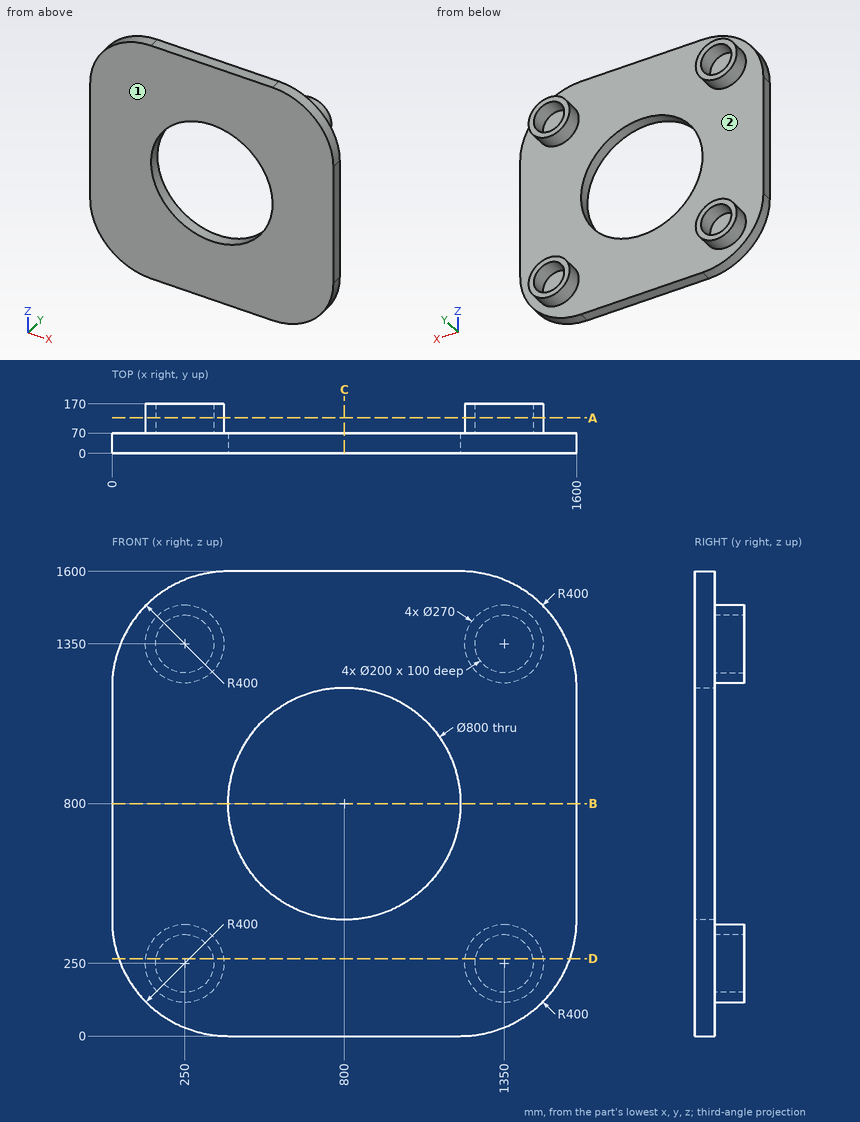
Geometry: see drawing. Coordinates: mm, zero at the bounding-box minimum. Coordinates: 2 decimals unless noted, no trailing zeros. Loops run counter-clockwise (first coordinate to the right, second up) from the corner with the lowest first, then second, coordinate; pieces in that order, holes last. Notation, with made-up numbers: (6, 87) -> (26, 87) arc R18 cw to (26, 118) -> close; hole circle Ø3 at (69, 64.5). An arc over 180 degrees is marked (long way). Use a Markdown table: item, result.
1) Cut plane C-C (x = 800). Return the cut outline in (y, z).
Results found:
| item | result |
|---|---|
| outline | (0, 0) -> (70, 0) -> (70, 400) -> (0, 400) -> close; (0, 1200) -> (70, 1200) -> (70, 1600) -> (0, 1600) -> close |
2) Cut plane D-D (z = 266.5). Return the cut outline in (x, y), then the cut area to 3 significant figures.
Results found:
| item | result |
|---|---|
| outline | (22.94, 0) -> (1577.06, 0) -> (1577.06, 70) -> (1483.99, 70) -> (1483.99, 170) -> (1448.63, 170) -> (1448.63, 70) -> (1251.37, 70) -> (1251.37, 170) -> (1216.01, 170) -> (1216.01, 70) -> (383.99, 70) -> (383.99, 170) -> (348.63, 170) -> (348.63, 70) -> (151.37, 70) -> (151.37, 170) -> (116.01, 170) -> (116.01, 70) -> (22.94, 70) -> close |
| area | 123,000 mm2 |
3) Cut plane A-A (y = 122). Return the cut outline in (x, z).
Results found:
| item | result |
|---|---|
| outline | circle Ø270 at (250, 250); circle Ø270 at (250, 1350); circle Ø270 at (1350, 250); circle Ø270 at (1350, 1350); hole circle Ø200 at (250, 250); hole circle Ø200 at (250, 1350); hole circle Ø200 at (1350, 250); hole circle Ø200 at (1350, 1350) |
4) Cut plane B-B (z = 800). Return the cut outline in (x, y), then the cut area to 3 significant figures.
Results found:
| item | result |
|---|---|
| outline | (0, 0) -> (400, 0) -> (400, 70) -> (0, 70) -> close; (1200, 0) -> (1600, 0) -> (1600, 70) -> (1200, 70) -> close |
| area | 56,000 mm2 |
5) Pull-direction query (X, two-part tool) for the marked faces 1 and 2; classes: released by +X, released by -X, zero draft, split by the parting line, or undercut.
Results found:
| item | result |
|---|---|
| face 1 | zero draft |
| face 2 | undercut |
6) Contact query for flat-ended pins moving along their axis: pin 1 (1 mm diameter, centred on y = 93, z = 1242, fed in from -X); pin 2 (10 mm diameter, centred on y = 107.5, z = 1313, fed in from -X); pin 3 (12 mm diameter, centred on x = 1222.5, y = 117.5, fed in from -Z). Output: stop coordinate, or through.
Results found:
| item | result |
|---|---|
| pin 1 | stops at x = 168.34 |
| pin 2 | stops at x = 118.85 |
| pin 3 | stops at z = 191.15 |
7) Material intervals for line 1 along X through (y, z) = (128, 1350); line 2 along Z through (x, y) = (1375, 74) (3 decimals); line 3 along X through (y, z) = (98, 268), sorted ascending. Write a range as from..to.
Results found:
| item | result |
|---|---|
| line 1 | x = 115..150, 350..385, 1215..1250, 1450..1485 |
| line 2 | z = 117.335..153.175, 346.825..382.665, 1217.335..1253.175, 1446.825..1482.665 |
| line 3 | x = 116.21..151.63, 348.37..383.79, 1216.21..1251.63, 1448.37..1483.79 |
